Geometry: see drawing. Coordinates: mm, zero at the bounding-box minimum. A direction names the side the tool comes from. Coordinates: 2 decimals unless noted, no trailing zeros. Loops run counter-clockwise (first coordinate to the right, second up) from the corner with the lowest first, then second, coordinate; pieces in that order, holes last. Notation, with made-up numbers: (-20.75, 36) - (-1.75, 36) arc R32 ccw to (-1.75, 75) - close; hole circle Ø5 at (14.25, -37.75). An arc over 180 degrees is marked (long way). Use a Markdown table: item, result. Add a question column.
1. Section query C-C on z = 3. State how many separate pieces and enclosed holes the cut face has, then the cut area to 3 significant figures.
2. Section query B-B on y = 30. Return the cut outline in (x, z).
3. Access query for the marked faces 1 and 2. Directions: +Z, -Z, +X, -X, +Y, -Y. A direction counts if a zero-diameter tool reaches every point of the face in a straight line with its end or side. Return the directions, or none.
4. Ray query, L1, parallel to Y at x = 10, z = 2.5; L2, parallel to X at y = 29.5, z = 11.5; L3, parallel to Y at x = 90, z = 5. Return the intervals inside material, ascending. Write a range as [from, to].
5. Section query A-A on x = 10. Return the cut outline in (y, z), then the cut area to 3 significant figures.
6. Section query D-D on x = 90. Return the cut outline in (y, z).
7. Contact query for flat-ended pins moving along their axis: P1, Ø6.5, axis at x = 10, y = 10, coming from the +Z side; P2, Ø3.5, axis at x = 140, z = 8, coming from the -Y side; P3, Ø13, axis at x = 90, y = 30, coming from the +Z side; P4, Ø4, axis at x = 25.5, z = 10, coming from the -Y side. Output: stop coordinate, or through.
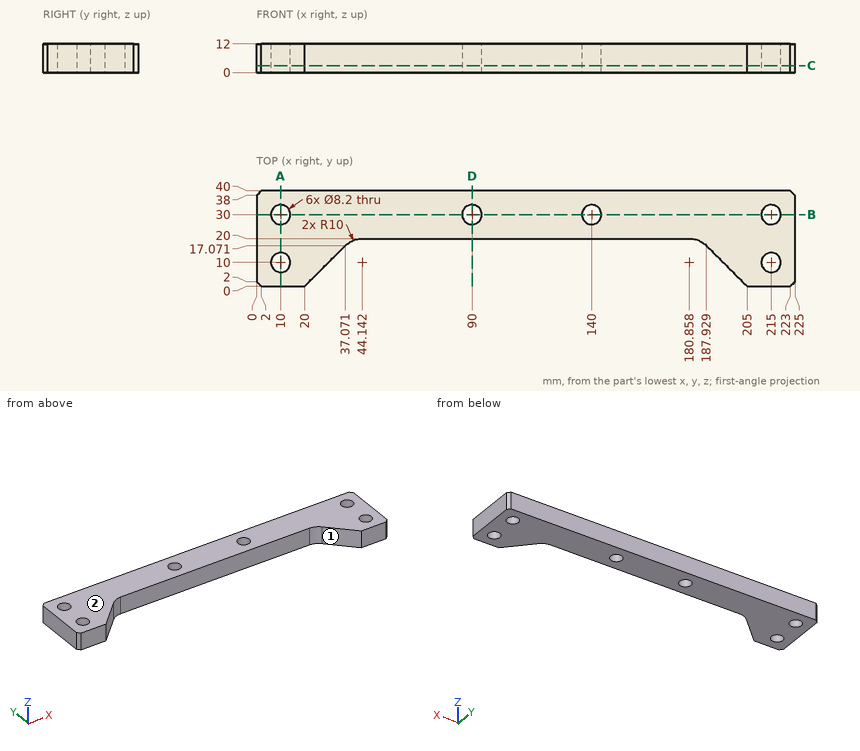
Resolved:
| question | item | result |
|---|---|---|
| 1 | separate pieces | 1 |
| 1 | enclosed holes | 6 |
| 1 | area | 5,380 mm² |
| 2 | outline | (0, 0) - (5.9, 0) - (5.9, 12) - (0, 12) - close; (14.1, 0) - (85.9, 0) - (85.9, 12) - (14.1, 12) - close; (94.1, 0) - (135.9, 0) - (135.9, 12) - (94.1, 12) - close; (144.1, 0) - (210.9, 0) - (210.9, 12) - (144.1, 12) - close; (219.1, 0) - (225, 0) - (225, 12) - (219.1, 12) - close |
| 3 | face 1 | +Z, -Z, -Y |
| 3 | face 2 | +Z, +X, -X, +Y, -Y |
| 4 | L1 | [0, 5.9], [14.1, 25.9], [34.1, 40] |
| 4 | L2 | [0, 5.93], [14.07, 85.93], [94.07, 135.93], [144.07, 210.93], [219.07, 225] |
| 4 | L3 | [20, 25.9], [34.1, 40] |
| 5 | outline | (0, 0) - (5.9, 0) - (5.9, 12) - (0, 12) - close; (14.1, 0) - (25.9, 0) - (25.9, 12) - (14.1, 12) - close; (34.1, 0) - (40, 0) - (40, 12) - (34.1, 12) - close |
| 5 | area | 283 mm² |
| 6 | outline | (20, 0) - (25.9, 0) - (25.9, 12) - (20, 12) - close; (34.1, 0) - (40, 0) - (40, 12) - (34.1, 12) - close |
| 7 | P1 | through |
| 7 | P2 | y = 20 |
| 7 | P3 | z = 12 |
| 7 | P4 | y = 3.5 |
